Check sheet for the modelled part. Datum: model origin and axes. Units: mm. A direction names the side the tool comes from. Give positions to 0.01 mm unless a question says otherwise; leave off trailing zeros. Write each loop counter-clockwise with the first axis right and the second up, starting at its lowest first coordinate (ties: lowest second). Pieces come first, ordered by that corner, then holes. Notation, with made-up numbers: (37.5, 29.5) -> (73.5, 29.5) arc R18 ccw to (73.5, 56.5) -> close; hole circle Ø11 at (33, 50.5). An arc over 180 degrees is marked (long way). Return JSON: item names as keys, results as strings.
from build123d import *

# Parameters (mm, degrees)
BOSS_EXTRUDE1_DEPTH = 78
SKETCH4_R           = 16
BOSS_EXTRUDE2_DEPTH = 3
SKETCH5_R           = 4
BOSS_EXTRUDE3_DEPTH = 16.4
SKETCH7_R           = 2
CUT_EXTRUDE2_DEPTH  = 9
SKETCH8_R           = 2
CUT_EXTRUDE3_DEPTH  = 10
SKETCH9_R           = 2.5
CUT_EXTRUDE4_DEPTH  = 10


with BuildPart() as part:
    # Sketch3 → Boss-Extrude1 (new body)
    with BuildSketch(Plane.XY):
        with BuildLine():
            Line((-16, -20), (16, -20))
            ThreePointArc((16, -20), (18.828427125, -18.828427125), (20, -16))
            Line((20, -16), (20, 16))
            ThreePointArc((20, 16), (18.828427125, 18.828427125), (16, 20))
            Line((16, 20), (-16, 20))
            ThreePointArc((-16, 20), (-18.828427125, 18.828427125), (-20, 16))
            Line((-20, 16), (-20, -16))
            ThreePointArc((-20, -16), (-18.828427125, -18.828427125), (-16, -20))
        make_face()
    extrude(amount=BOSS_EXTRUDE1_DEPTH)

    # Sketch4 → Boss-Extrude2 (add)
    with BuildSketch(Plane(origin=(0, 0, 0), x_dir=(-1, 0, 0), z_dir=(0, 0, -1))):
        Circle(SKETCH4_R)
    extrude(amount=BOSS_EXTRUDE2_DEPTH)

    # Sketch5 → Boss-Extrude3 (add)
    with BuildSketch(Plane(origin=(0, 0, -3), x_dir=(-1, 0, 0), z_dir=(0, 0, -1))):
        Circle(SKETCH5_R)
    extrude(amount=BOSS_EXTRUDE3_DEPTH)

    # Sketch7 → Cut-Extrude2 (cut)
    with BuildSketch(Plane(origin=(0, 0, 0), x_dir=(-1, 0, 0), z_dir=(0, 0, -1))):
        with Locations((-15.5, 15.5)):
            Circle(SKETCH7_R)
        with Locations((15.5, 15.5)):
            Circle(SKETCH7_R)
        with Locations((15.5, -15.5)):
            Circle(SKETCH7_R)
        with Locations((-15.5, -15.5)):
            Circle(SKETCH7_R)
    extrude(amount=-CUT_EXTRUDE2_DEPTH, mode=Mode.SUBTRACT)

    # Sketch8 → Cut-Extrude3 (cut)
    with BuildSketch(Plane.XY.offset(78)):
        with Locations((-16, 8)):
            Circle(SKETCH8_R)
        with Locations(Location((16, 8, 0), (0, 0, 180))):
            Circle(SKETCH8_R)
        with Locations(Location((-16, -8, 0), (0, 0, 180))):
            Circle(SKETCH8_R)
        with Locations((16, -8)):
            Circle(SKETCH8_R)
    extrude(amount=-CUT_EXTRUDE3_DEPTH, mode=Mode.SUBTRACT)

    # Sketch9 → Cut-Extrude4 (cut)
    with BuildSketch(Plane.XY.offset(78)):
        with Locations((10, 0)):
            Circle(SKETCH9_R)
        with Locations(Location((-10, 0, 0), (0, 0, 180))):
            Circle(SKETCH9_R)
    extrude(amount=-CUT_EXTRUDE4_DEPTH, mode=Mode.SUBTRACT)


solid = part.part
(1) Cross-section at B-B on y = 0. Enter the section's corners in (x, z).
Reply:
{"outline": "(-20, 0) -> (-16, 0) -> (-16, -3) -> (-4, -3) -> (-4, -19.4) -> (4, -19.4) -> (4, -3) -> (16, -3) -> (16, 0) -> (20, 0) -> (20, 78) -> (12.5, 78) -> (12.5, 68) -> (7.5, 68) -> (7.5, 78) -> (-7.5, 78) -> (-7.5, 68) -> (-12.5, 68) -> (-12.5, 78) -> (-20, 78) -> close"}
(2) Cross-section at D-D on y = -11. Enter the section's corners in (x, z), then the cut area to 3 significant figures.
Reply:
{"outline": "(-20, 0) -> (-11.62, 0) -> (-11.62, -3) -> (11.62, -3) -> (11.62, 0) -> (20, 0) -> (20, 78) -> (-20, 78) -> close", "area": "3,190 mm^2"}
(3) Set-up check for faces 4 (the flat face through (10, 0, 68)), 5 (the flat face through (-3, -3, -3)), 6 (the flat face through (0, 0, -19.4)): record each of +Z, -Z, +X, -X, +Y, -Y from which the full face is reachable in a straight line by a thin tool's end or side.
Reply:
{"face 4": "+Z", "face 5": "-Z", "face 6": "-Z, +X, -X, +Y, -Y"}
(4) Thickness scan on L1, parallel to Y at x = 16, z = 71.25; L2, parallel to Y at x = -10, z = 76.25; L3, parallel to X at y = -15, z = 5. Record the ranges inside material, lowest first.
Reply:
{"L1": "-20 to -10, -6 to 6, 10 to 20", "L2": "-20 to -2.5, 2.5 to 20", "L3": "-20 to -17.44, -13.56 to 13.56, 17.44 to 20"}
(5) Cross-section at A-A on x = 0. Enter the section's corners in (y, z), then the cut area to 3 significant figures.
Reply:
{"outline": "(-20, 0) -> (-16, 0) -> (-16, -3) -> (-4, -3) -> (-4, -19.4) -> (4, -19.4) -> (4, -3) -> (16, -3) -> (16, 0) -> (20, 0) -> (20, 78) -> (-20, 78) -> close", "area": "3,350 mm^2"}
(6) Release check for a two-part mould opening along Y. For faces 1 (the cylindrical face through (18.859, 18.797, 38.454)), 2 (the cylindrical face through (-17.474, 9.352, 73.07)), 3 (the flat face through (0, -20, 38)) record: pulls with the +Y half, pulls with the -Y half, needs draft (parallel to the pull), parting line crosses it, or undercut.
Reply:
{"face 1": "pulls with the +Y half", "face 2": "undercut", "face 3": "pulls with the -Y half"}
(7) Cross-section at C-C on x = -11. Enter the section's corners in (y, z), then the cut area to 3 significant figures.
Reply:
{"outline": "(-20, 0) -> (-11.62, 0) -> (-11.62, -3) -> (11.62, -3) -> (11.62, 0) -> (20, 0) -> (20, 78) -> (2.29, 78) -> (2.29, 68) -> (-2.29, 68) -> (-2.29, 78) -> (-20, 78) -> close", "area": "3,140 mm^2"}
(8) Depth check by flat-ended pin: pin 1 Ø1.2 at (x, y) = (15.5, -7.5) entering from +Z; pin 2 Ø1.2 at (x, y) = (-15.5, 14.5) entering from -Z; pin 3 Ø6 at (x, z) = (6, -4.5) entering from +Y. Enter the tip coordinate at first touch or a pass-through.
Reply:
{"pin 1": "z = 68", "pin 2": "z = 9", "pin 3": "y = 15.63"}
